Can you work these out from the model? Positions are in its coordinate system, mm. Give positions to 0.01 mm unless a question says otherwise; leave off trailing zeros. Write each loop counter-clockwise with the first axis right and the second up, starting at its lowest first coordinate (ties: lowest second). Pieces come first, ordered by that corner, then holes.
1. Suppose I cut it at A-A (x = 2.5). Please give me the cut outline in (y, z).
2. I'm going to push a flat-ended pin straight in: pin 1 (2 mm diameter, centred on x = 8.5, z = -0.5, fed in from +Y). Where does the tip first touch, or does it pass through?
3. If I drill on probe 1 along Y at (x, z) = (0.5, -0.25); probe 2 along Y at (x, z) = (1, -0.7); probe 3 along Z at (x, y) = (13, 0.9), over which ranges is the centre line in solid material (lowest first)?
```python
from build123d import *

# Parameters (mm, degrees)
RECPAT_COUNT    = 2
RECPAT_ANGLE    = 90
THDSCHPAT_COUNT = 26
THDSCHPAT_PITCH = 0.444


with BuildPart() as part:
    # Fillet1: read off the stored shape, not the designer's step
    # Fillet1 outline → Fillet1 (revolve)
    with BuildSketch(Plane.YX):
        with BuildLine():
            Line((1.25, 2.2), (1.25, 14.1))
            Line((1.25, 14.1), (0, 14.1))
            Line((0, 14.1), (0, 0))
            ThreePointArc((0, 0), (1.267435139, 0.206109099), (2.404255321, 0.803195916))
            ThreePointArc((2.404255321, 0.803195916), (2.474733878, 0.88781572), (2.5, 0.99500416))
            Line((2.5, 0.99500416), (2.5, 2.1))
            Line((2.5, 2.1), (1.35, 2.1))
            ThreePointArc((1.35, 2.1), (1.279289322, 2.129289322), (1.25, 2.2))
        make_face()
    revolve(axis=Axis((0, 0, 0), (1, 0, 0)))

    # Sketch3 → Recess section 0
    with BuildSketch(Plane(origin=(0, 0, 0), x_dir=(0, 0, -1), z_dir=(1, 0, 0))):
        with BuildLine():
            Line((0.37, -1.3), (-0.37, -1.3))
            Line((-0.37, -1.3), (-0.37, 1.3))
            Line((-0.37, 1.3), (0.37, 1.3))
            Line((0.37, 1.3), (0.37, -1.3))
        make_face()
    # Sketch4 → Recess section 1
    with BuildSketch(Plane(origin=(1.5, 0, 0), x_dir=(0, 0, -1), z_dir=(1, 0, 0))):
        with BuildLine():
            Line((0.37, -0.552127713), (-0.37, -0.552127713))
            Line((-0.37, -0.552127713), (-0.37, 0.552127713))
            Line((-0.37, 0.552127713), (0.37, 0.552127713))
            Line((0.37, 0.552127713), (0.37, -0.552127713))
        make_face()
    recess = loft(mode=Mode.SUBTRACT)

    # RecPat: Recess ×2 about axis
    recpat_axis = Axis((0, 0, 0), (1, 0, 0))
    for i in range(1, RECPAT_COUNT):
        add(recess.rotate(recpat_axis, i * RECPAT_ANGLE / (RECPAT_COUNT - 1)), mode=Mode.SUBTRACT)

    # RecCorSke → RecessCore (revolve, cut)
    with BuildSketch(Plane.XY, mode=Mode.PRIVATE) as recesscore_sk:
        Polygon((0, 0), (0, 0.660890218), (1.5, 0.556), (1.680655351, 0), align=None)
    revolve(recesscore_sk.sketch.rotate(Axis((-3.175, 0, 0), (1, 0, 0)), 90), axis=Axis((-3.175, 0, 0), (1, 0, 0)), mode=Mode.SUBTRACT)

    # ThdSchSke → ThreadSchematic (revolve, cut)
    with BuildSketch(Plane.XY, mode=Mode.PRIVATE) as threadschematic_sk:
        Polygon((3, -0.9965), (2.822497389, -1.25), (2.822497389, -1.5625), (3.177502611, -1.5625), (3.177502611, -1.25), align=None)
    threadschematic = revolve(threadschematic_sk.sketch.rotate(Axis((-3.175, 0, 0), (1, 0, 0)), 270), axis=Axis((-3.175, 0, 0), (1, 0, 0)), mode=Mode.SUBTRACT)

    # ThdSchPat: ThreadSchematic ×26
    with Locations(*[(i * THDSCHPAT_PITCH, 0, 0) for i in range(1, THDSCHPAT_COUNT)]):
        add(threadschematic, mode=Mode.SUBTRACT)


solid = part.part
```
Checks:
1. outline: circle Ø2.5 at (0, 0)
2. pin 1: stops at y = 1.25
3. probe 1: y = -1.92 to -1.05, 1.05 to 1.92
3. probe 2: y = -2.4 to -0.37, 0.37 to 2.4
3. probe 3: z = -0.87 to 0.87
